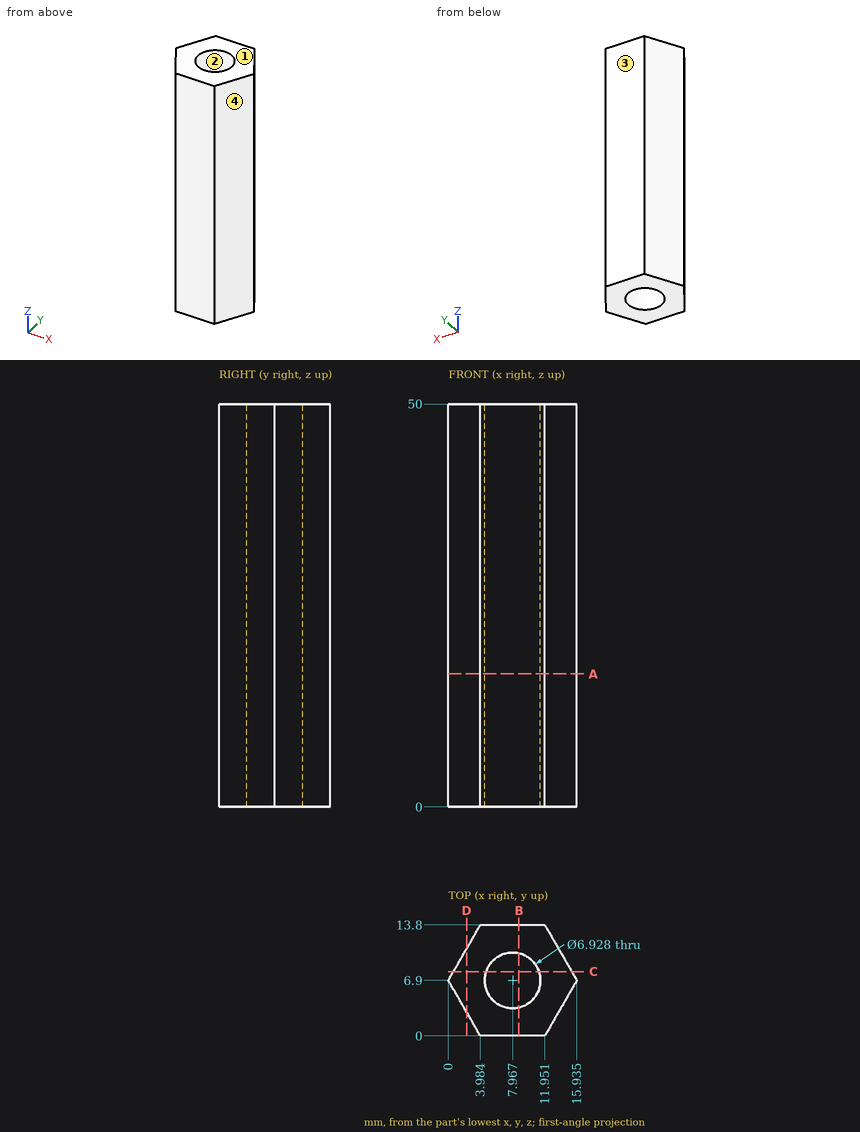
Could you check a few things on this drawing? It's one solid part, dimensions in mm from its lowest x, y, z. Coordinates: 2 decimals unless noted, no trailing zeros. Order: outer loops, then holes, each group sorted by start corner. A loop starts at its lowest first (then second) coordinate and runs counter-clockwise, first axis right, second up. Notation, with made-up numbers: (86, 62.5) - (99, 62.5) arc R5 cw to (99, 68.5) - close; hole circle Ø8 at (6.25, 8). An arc over 180 degrees is marked (long way). One line per question, with ' | ' between items. Start each with the question number.
1. If we mould it in two halves opening along Y, with no side actions, what happens to the marked faces 1, 2, 3 and 4? For each: released by +Y, released by -Y, zero draft, split by the parting line, or undercut.
2. If we section it at B-B (x = 8.75): Write out the boundary of the cut face in (y, z) (1 decimal).
3. Please list where these lines run through material, in increasing order: line 1 along X through (y, z) = (9, 8); line 2 along Y through (x, z) = (6.5, 31); line 3 along X through (y, z) = (5.25, 22) (1 decimal). Write a range as [from, to].
4. If we section it at A-A (z = 16.5): Write out the boundary of the cut face in (x, y) (1 decimal).
5. I'm going to push flat-ended pins straight in: pin 1 Ø1 at (y, z) = (9.5, 9) entering from +X; pin 2 Ø3 at (y, z) = (5, 30) entering from -X; pin 3 Ø1 at (y, z) = (3, 39.5) entering from -X. Where does each tip first touch, or does it pass through?
6. If we section it at C-C (y = 8): Write out the boundary of the cut face in (x, z) (1 decimal), and give its area (3 significant figures).
7. If we section it at D-D (x = 2.25): Write out the boundary of the cut face in (y, z), and give its area (3 significant figures).
Model answer:
1) face 1: zero draft | face 2: undercut | face 3: released by +Y | face 4: released by -Y
2) outline: (0, 0) - (3.5, 0) - (3.5, 50) - (0, 50) - close; (10.3, 0) - (13.8, 0) - (13.8, 50) - (10.3, 50) - close
3) line 1: x = [1.21, 5.21], [10.72, 14.72] | line 2: y = [0, 3.76], [10.04, 13.8] | line 3: x = [1, 4.9], [11, 15]
4) outline: (0, 6.9) - (4, 0) - (12, 0) - (15.9, 6.9) - (12, 13.8) - (4, 13.8) - close; hole circle Ø6.9 at (8, 6.9)
5) pin 1: stops at x = 14.72 | pin 2: stops at x = 0.23 | pin 3: stops at x = 1.96
6) outline: (0.6, 0) - (4.7, 0) - (4.7, 50) - (0.6, 50) - close; (11.3, 0) - (15.3, 0) - (15.3, 50) - (11.3, 50) - close | area: 405 mm²
7) outline: (3, 0) - (10.8, 0) - (10.8, 50) - (3, 50) - close | area: 390 mm²
